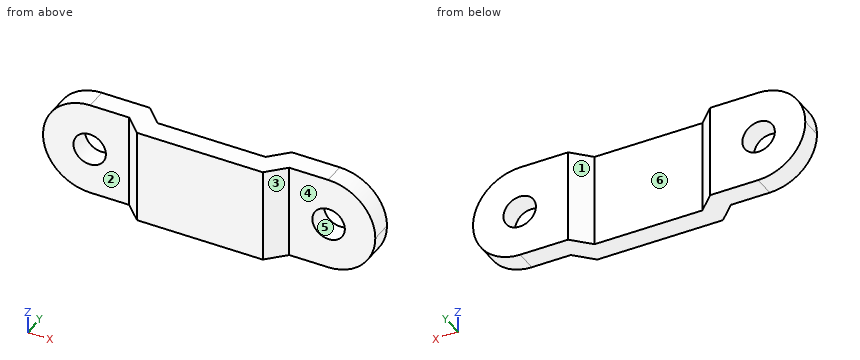
from build123d import *

# Parameters (mm, degrees)
BASE_EXTRUDE_DEPTH = 11.0744
SKETCH2_R          = 1.905
CUT_EXTRUDE1_DEPTH = 23.889284907
FILLET1_R          = 5.5372


with BuildPart() as part:
    # Sketch1 → Base-Extrude (new body)
    with BuildSketch(Plane.XY):
        Polygon((-8.342087552, -2.54), (-6.330407552, -4.55168), (6.330407552, -4.55168), (8.342087552, -2.54), (19.507927552, -2.54), (19.507927552, -5.08), (9.39419, -5.08), (7.38251, -7.09168), (-7.38251, -7.09168), (-9.39419, -5.08), (-19.507927552, -5.08), (-19.507927552, -2.54), align=None)
    extrude(amount=BASE_EXTRUDE_DEPTH)

    # Sketch2 → Cut-Extrude1 (cut, through all)
    with BuildSketch(Plane(origin=(0, -2.54, 0), x_dir=(-1, 0, 0), z_dir=(0, 1, 0))):
        with Locations((14.026607552, 5.481627302)):
            Circle(SKETCH2_R)
    cut_extrude1 = extrude(amount=-CUT_EXTRUDE1_DEPTH, mode=Mode.SUBTRACT)

    # Mirror1: Cut-Extrude1 across plane
    add(cut_extrude1.mirror(Plane(origin=(0, 0, 0), x_dir=(0, 0, 1), z_dir=(1, 0, 0))), mode=Mode.SUBTRACT)

    # Fillet1
    fillet1_edges = [part.edges().sort_by_distance(p)[0] for p in [
        (19.507927552, -3.81, 0),
        (-19.507927552, -3.81, 0),
        (19.507927552, -3.81, 11.0744),
        (-19.507927552, -3.81, 11.0744),
    ]]
    fillet(fillet1_edges, radius=FILLET1_R - 0.0001)  # a hair under: the kernel refuses the full size


solid = part.part
CAD build for the part. Positions are in the model's coordinates, mm. Face numbers are marked on the shaded views. A direction names the side the tool comes from. Coordinates: 2 decimals unless noted, no trailing zeros. Loops run counter-clockwise (first coordinate to the right, second up) from the corner with the lowest first, then second, coordinate; pieces in that order, holes last. Notation, with made-up numbers: (-26.5, -26.75) - (26.5, -26.75) arc R27 cw to (26.5, 7.25) - close; hole circle Ø3 at (-12.75, 57). An arc over 180 degrees is marked (long way). Write item = value, one per line. Start each with the question number.
Q1. Which spindle directions (+Z, -Z, +X, -X, +Y, -Y) get a long thin tool onto all of the face, cutting with end or side? Do the marked faces 4, 5 and 6. Say none if no direction does.
Q2. Cut at C-C, the plane z = 3.25. List the corners of the cut face in (x, y).
Q3. Drill centre lines: L1, parallel to Y at x = 14, z = 9.75; L2, parallel to X at y = -3.3, z = 6.25; L3, parallel to Z at x = 14.5, y = -3.1. Where is each one in solid material? Low to high.
Q4. Pull direction X, two halves, no side cores. Call the marked faces 1, 2 and 3: pulls with the +X half, pulls with the -X half, needs draft (parallel to the pull), parting line crosses it, or undercut.
Q5. Flat gauge pins, fed straight in: pin 1 Ø5 at (x, z) = (15.5, 5) entering from -Y; pin 2 Ø1 at (y, z) = (-4.5, 7.5) entering from +X; pin 3 Ø1.5 at (y, z) = (-3.5, 7) entering from -X. Where does each tip first touch, or does it go through?
Q6. Cut at D-D, the plane x = 11. List the corners of the cut face in (y, z), then the cut area to 3 significant figures.
Q7. Cut at A-A, the plane y = -3.75. Give the number of separate pieces and of enclosed holes in the cut face, then the cut area to 3 significant figures.
Q8. Cut at B-B, the plane z = 4.75. List the corners of the cut face in (x, y), then the cut area to 3 significant figures.
Computed:
q1.face_4 = +Z, -Z, +X, -Y
q1.face_5 = +Y, -Y
q1.face_6 = +Z, -Z, +Y
q2.outline = (-19.01, -5.08) - (-9.39, -5.08) - (-7.38, -7.09) - (7.38, -7.09) - (9.39, -5.08) - (19.01, -5.08) - (19.01, -2.54) - (8.34, -2.54) - (6.33, -4.55) - (-6.33, -4.55) - (-8.34, -2.54) - (-19.01, -2.54) - close
q3.L1 = -5.08 to -2.54
q3.L2 = -19.46 to -15.77, -12.28 to -7.58, 7.58 to 12.28, 15.77 to 19.46
q3.L3 = 0.03 to 3.64, 7.33 to 11.05
q4.face_1 = undercut
q4.face_2 = needs draft
q4.face_3 = pulls with the +X half
q5.pin_1 = -5.08
q5.pin_2 = 19.31
q5.pin_3 = -19.46
q6.outline = (-5.08, 0) - (-2.54, 0) - (-2.54, 11.07) - (-5.08, 11.07) - close
q6.area = 28.1 mm²
q7.separate_pieces = 2
q7.enclosed_holes = 2
q7.area = 225 mm²
q8.outline = (-19.45, -5.08) - (-15.79, -5.08) - (-15.79, -2.54) - (-19.45, -2.54) - close; (-12.27, -5.08) - (-9.39, -5.08) - (-7.38, -7.09) - (7.38, -7.09) - (9.39, -5.08) - (12.27, -5.08) - (12.27, -2.54) - (8.34, -2.54) - (6.33, -4.55) - (-6.33, -4.55) - (-8.34, -2.54) - (-12.27, -2.54) - close; (15.79, -5.08) - (19.45, -5.08) - (19.45, -2.54) - (15.79, -2.54) - close
q8.area = 85.2 mm²
